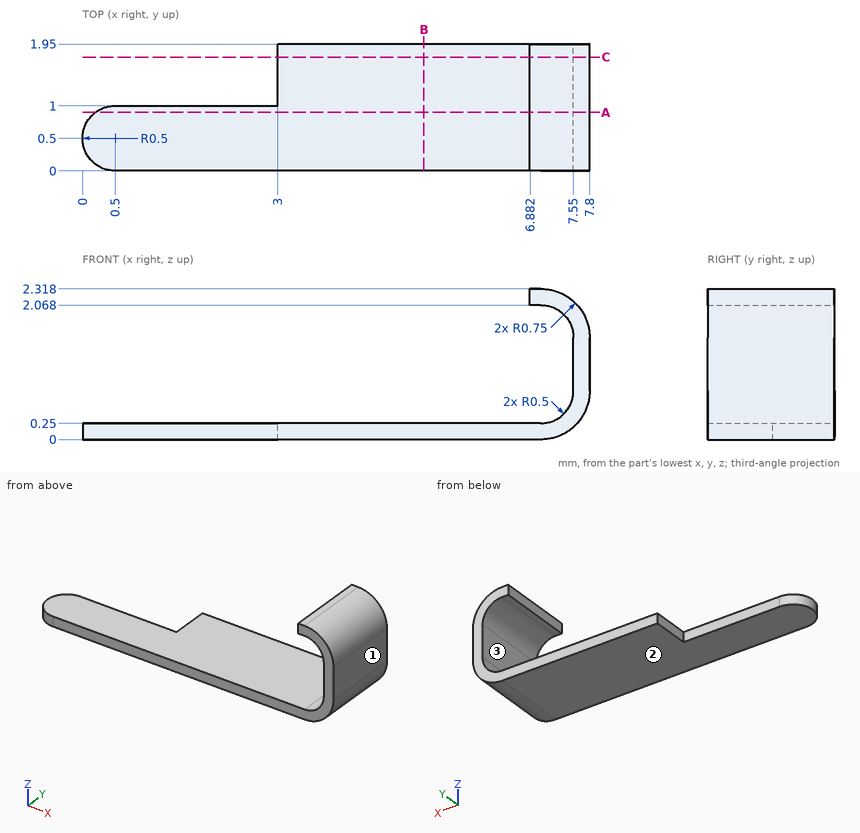
The drawing under review shows one solid part. Ordinate dimensions are in mm from its lowest x, y, z. Round coordinates to 2 decimals unless told otherwise and drop trailing zeros. Loops run counter-clockwise (first coordinate to the right, second up) from the corner with the lowest first, then second, coordinate; pieces in that order, holes last. Notation, with made-up numbers: (50.5, 28) - (89.5, 28) arc R20 ccw to (89.5, 41) - close; hole circle Ø2 at (31.5, 73.5). An arc over 180 degrees is marked (long way). Use one line per item in the form item = value.
Item 1: Clearance check with flat-ended pins moving along their axes: P1, Ø1, axis at y = 0.5, z = 2, coming from the -X side; P2, Ø1, axis at x = 2, y = 0.5, coming from the +Z side; P3, Ø1, axis at x = 5, z = 1.5, coming from the +Y side. State where each tip first meets the part, or that it passes through.
Answers:
P1 = 6.88
P2 = 0.25
P3 = through
Item 2: Mouldability with a two-part tool opening along Z and no side actions: class the marked faces 1, 2 and 3 as +Z half, -Z half, draft (parallel to the pull), parting line (faces both ways), or undercut.
Answers:
face_1 = draft
face_2 = -Z half
face_3 = undercut
Item 3: Consider section A-A on y = 0.9. Write out the cut boundary in (x, z).
Answers:
outline = (0.2, 0) - (7.05, 0) arc R0.75 ccw to (7.8, 0.75) - (7.8, 1.57) arc R0.75 ccw to (7.05, 2.32) - (6.88, 2.32) - (6.88, 2.07) - (7.05, 2.07) arc R0.5 cw to (7.55, 1.57) - (7.55, 0.75) arc R0.5 cw to (7.05, 0.25) - (0.2, 0.25) - close
Item 4: Consider section C-C on y = 1.75. Write out the cut boundary in (x, z).
Answers:
outline = (3, 0) - (7.05, 0) arc R0.75 ccw to (7.8, 0.75) - (7.8, 1.57) arc R0.75 ccw to (7.05, 2.32) - (6.88, 2.32) - (6.88, 2.07) - (7.05, 2.07) arc R0.5 cw to (7.55, 1.57) - (7.55, 0.75) arc R0.5 cw to (7.05, 0.25) - (3, 0.25) - close
Item 5: For line 1 (Z direction, x = 7, y = 0.1); line 2 (Z direction, x = 3.75, y = 0.6), list the stretches that pass through material, from the lowest coordinate up.
Answers:
line_1 = 0 to 0.25, 2.07 to 2.32
line_2 = 0 to 0.25
Item 6: Consider section B-B on x = 5.25. Write out the cut boundary in (y, z).
Answers:
outline = (0, 0) - (1.95, 0) - (1.95, 0.25) - (0, 0.25) - close
